```python
from build123d import *

# Parameters (mm, degrees)
F0_W      = 60.821578
F0_H      = 104.845289
F1_DEPTH  = 2.54
F2_R      = 5.08
F3_R      = 5.08
F4_R      = 5.08
F5_R      = 5.08
F6_R      = 4.017184
F7_DEPTH  = 0.762
F8_W      = 20.353574
F8_H      = 6.179251
F9_DEPTH  = 0.762
F10_R     = 1.27
F11_W     = 52.752584
F11_H     = 85.154727
F12_DEPTH = 2.045468
F13_W     = 50.705392
F13_H     = 3.825493
F14_DEPTH = 0.505788
F16_R     = 1.146481
F17_DEPTH = 1.574736
F19_W     = 1.183123
F19_H     = 12.295741
F20_DEPTH = 0.381
F21_W     = 1.133876
F21_H     = 11.616781
F22_DEPTH = 0.540292


with BuildPart() as f1:
    # F0 (on Front) → F1 (new body)
    with BuildSketch(Plane.XZ):
        with Locations((-0.1534, -3.119452)):
            Rectangle(F0_W, F0_H)
    extrude(amount=F1_DEPTH)

    # F2
    f2_edges = [f1.edges().sort_by_distance(p)[0] for p in [
        (30.257389, -1.27, -55.542096),
    ]]
    fillet(f2_edges, radius=F2_R)

    # F3
    f3_edges = [f1.edges().sort_by_distance(p)[0] for p in [
        (-30.564189, -1.27, -55.542096),
    ]]
    fillet(f3_edges, radius=F3_R)

    # F4
    f4_edges = [f1.edges().sort_by_distance(p)[0] for p in [
        (-30.564189, -1.27, 49.303193),
    ]]
    fillet(f4_edges, radius=F4_R)

    # F5
    f5_edges = [f1.edges().sort_by_distance(p)[0] for p in [
        (30.257389, -1.27, 49.303193),
    ]]
    fillet(f5_edges, radius=F5_R)

    # F6 (on face) → F7 (join)
    with BuildSketch(Plane(origin=(0, 0, 0), x_dir=(-1, 0, 0), z_dir=(0, 1, 0))):
        with Locations((-18.701095, 42.867944)):
            Circle(F6_R)
    extrude(amount=F7_DEPTH)

    # F8 (on face) → F9 (join)
    with BuildSketch(Plane(origin=(0, 0, 0), x_dir=(-1, 0, 0), z_dir=(0, 1, 0))):
        with Locations((-1.897635, 43.139625)):
            Rectangle(F8_W, F8_H)
    extrude(amount=F9_DEPTH)

    # F10
    f10_edges = [f1.edges().sort_by_distance(p)[0] for p in [
        (-8.279152, 0.381, 46.229251),
        (-8.279152, 0.381, 40.05),
        (12.074422, 0.381, 40.05),
        (12.074422, 0.381, 46.229251),
    ]]
    fillet(f10_edges, radius=F10_R)

    # F11 (on face) → F12 (cut)
    with BuildSketch(Plane.XZ.offset(2.54)):
        with Locations((0, -5.289763)):
            Rectangle(F11_W, F11_H)
    extrude(amount=-F12_DEPTH, mode=Mode.SUBTRACT)

    # F13 (on face) → F14 (cut)
    with BuildSketch(Plane.XZ.offset(2.54)):
        with Locations((0.016911, -51.271375)):
            Rectangle(F13_W, F13_H)
    extrude(amount=-F14_DEPTH, mode=Mode.SUBTRACT)

    # F16 (on face) → F17 (cut)
    with BuildSketch(Plane.XY.offset(49.303193)):
        with Locations((18.786654, -1.340227)):
            Circle(F16_R)
    extrude(amount=-F17_DEPTH, mode=Mode.SUBTRACT)

    # F19 (on face) → F20 (join)
    with BuildSketch(Plane(origin=(-30.564189, 0, 0), x_dir=(0, -1, 0), z_dir=(-1, 0, 0))):
        with Locations((1.301603, 31.14997)):
            Rectangle(F19_W, F19_H)
    extrude(amount=F20_DEPTH)

    # F21 (on face) → F22 (join)
    with BuildSketch(Plane.YZ.offset(30.257389)):
        with Locations((-1.228773, 35.857343)):
            Rectangle(F21_W, F21_H)
    extrude(amount=F22_DEPTH)


solid = f1.part
```
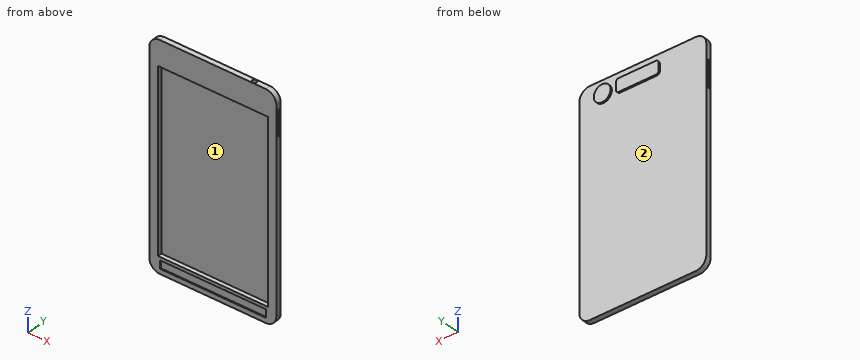
Verification items for the finished model (mm, model axes). Face numbers are marked on the shaded views. Coordinates: 2 decimals unless noted, no trailing zeros. Write each loop counter-clockwise with the first axis right and the second up, starting at its lowest first coordinate (ties: lowest second). Pieces come first, ordered by that corner, then holes. Notation, with made-up numbers: (4.25, 21.5) - (19.25, 21.5) arc R13 ccw to (19.25, 44.5) - close; hole circle Ø1 at (1, 9). An arc over 180 degrees is marked (long way). One line per question, with ' | ' between items. Start each with the question number.
1. Section check C-C (z = 0.5). Enter the section's corners in (x, y), plus the area to 3 significant figures.
2. Material ranges on line 1 along Z through (x, y) = (21, -2.35); line 2 along X through (y, z) = (-0.85, 12.5); line 3 along Z through (x, y) = (25.5, -2.1), recorded low to high.
3. Draft check along Z on the marked faces 1 and 2. Enter one of: released by +Z, released by -Z, zero draft, split by the parting line, or undercut.
4. Section check B-B (x = 13.5). Enter the section's corners in (y, z), plus the area to 3 significant figures.
5. Section check A-A (z = 32.5). Enter the section's corners in (x, y), plus the area to 3 significant figures.
6. Gauge pin test, flat ends, axial feed: P1, Ø0.8, axis at y = 0.5, z = 44, coming from the -X side; P2, Ø1.3, axis at y = -1, z = 19.5, coming from the -X side; P3, Ø2, axis at x = 11.5, z = 15.5, coming from the -Y side. Record the tip position at first contact, or that the pin passes through.
7. Section check D-D (x = 3). Enter the section's corners in (y, z), plus the area to 3 significant figures.
Computed values:
1) outline: (-30.56, -2.54) - (-26.38, -2.54) - (-26.38, -0.49) - (26.38, -0.49) - (26.38, -2.54) - (30.26, -2.54) - (30.26, 0) - (-30.56, 0) - close | area: 46.6 mm²
2) line 1: -55.54 to -53.18, -49.36 to -47.87, 37.29 to 49.3 | line 2: -30.56 to -26.38, 26.38 to 30.26 | line 3: -55.53 to -47.87, 37.29 to 49.29
3) face 1: undercut | face 2: zero draft
4) outline: (-2.54, -55.54) - (0, -55.54) - (0, 49.3) - (-2.54, 49.3) - (-2.54, 37.29) - (-0.49, 37.29) - (-0.49, -47.87) - (-2.54, -47.87) - (-2.54, -49.36) - (-2.03, -49.36) - (-2.03, -53.18) - (-2.54, -53.18) - close | area: 90.2 mm²
5) outline: (-30.95, -1.89) - (-30.56, -1.89) - (-30.56, -2.54) - (-26.38, -2.54) - (-26.38, -0.49) - (26.38, -0.49) - (26.38, -2.54) - (30.26, -2.54) - (30.26, -1.8) - (30.8, -1.8) - (30.8, -0.66) - (30.26, -0.66) - (30.26, 0) - (-30.56, 0) - (-30.56, -0.71) - (-30.95, -0.71) - close | area: 47.6 mm²
6) P1: x = -8.28 | P2: x = -30.56 | P3: y = -0.49
7) outline: (-2.54, -55.54) - (0, -55.54) - (0, 40.05) - (0.76, 40.05) - (0.76, 46.23) - (0, 46.23) - (0, 49.3) - (-2.54, 49.3) - (-2.54, 37.29) - (-0.49, 37.29) - (-0.49, -47.87) - (-2.54, -47.87) - (-2.54, -49.36) - (-2.03, -49.36) - (-2.03, -53.18) - (-2.54, -53.18) - close | area: 94.9 mm²
